Could you check a few things on this model? Use its own coordinates, in mm. A direction names the side the tool comes from. Round coordinates to 2 decimals unless told otherwise and drop trailing zeros. Order: outer loops, then holes, each group sorted by start corner. A loop starts at its lowest first (then second) coordinate and runs counter-clockwise, first axis right, second up. Notation, with made-up numbers: M 43,80.25 L 71,80.25 A24 cw 71,112.25 Z; hole C 39,62 d7. An arc over 180 degrees is marked long. Write each question's results on one line, items separated by ' | '. Start each with the question number.
1. Suppose I cut it at A-A on y = 946. Write out the boundary of the cut face in (x, z).
2. For faces 4 (the flat face through (-452, 553, 0)), 5 (the flat face through (-30, 276, 20)), which set-ups out of +Z, -Z, +X, -X, +Y, -Y let a thin tool reach every point of the face, with its end or its side?
3. Suppose I cut it at C-C on z = 28. Write out the boundary of the cut face in (x, y), and give its area (3 significant figures).
4. Suppose I cut it at B-B on x = -356.5. Write out the boundary of the cut face in (y, z).
5. We'd pull the mould along X, two halves only. Please class faces 1 (the flat face through (-870, 816, 20)), 2 (the flat face through (-19, 593, 50)), 3 (the flat face through (0, 542, 20)): released by +X, released by -X, zero draft, split by the parting line, or undercut.
6. I'm going to push flat-ended pins straight in: pin 1 (6 mm diameter, centred on x = -301, z = 50, fed in from +Y); pin 2 (5 mm diameter, centred on y = 542, z = 45, fed in from -X); pin 3 (6 mm diameter, centred on x = -693.5, z = 42.5, fed in from -Y); pin 4 (8 mm diameter, centred on y = 294, z = 45, fed in from -X). Where does each tip first touch, or does it pass through?
7. Please list where these lines run through material, in increasing order: L1, parallel to X at y = 1014, z = 35.5; L2, parallel to Y at x = -77, z = 37.5; L3, parallel to X at y = 364, z = 41.5.
from build123d import *

# Parameters (mm, degrees)
SKETCH1_W           = 900
SKETCH1_H           = 1100
SKETCH1_W_2         = 840
SKETCH1_H_2         = 1040
BOSS_EXTRUDE1_DEPTH = 50
FILLET1_R           = 10
SKETCH2_W           = 50
SKETCH2_H           = 1100
SKETCH2_W_2         = 868
SKETCH2_H_2         = 40
BOSS_EXTRUDE2_DEPTH = 60
FILLET2_R           = 10


with BuildPart() as part:
    # Sketch1 → Boss-Extrude1 (new body)
    with BuildSketch(Plane.XY):
        with Locations((-450, 550)):
            Rectangle(SKETCH1_W, SKETCH1_H)
        with Locations((-450, 550)):
            Rectangle(SKETCH1_W_2, SKETCH1_H_2, mode=Mode.SUBTRACT)
    extrude(amount=BOSS_EXTRUDE1_DEPTH)

    # Fillet1
    fillet1_edges = [part.edges().sort_by_distance(p)[0] for p in [
        (-900, 550, 50),
        (-450, 0, 50),
        (-450, 30, 50),
        (-30, 550, 50),
        (-450, 1070, 50),
        (-870, 550, 50),
        (0, 550, 50),
        (-450, 1100, 50),
    ]]
    fillet(fillet1_edges, radius=FILLET1_R)

    # Sketch2 → Boss-Extrude2 (add)
    with BuildSketch(Plane.XY):
        with Locations((-450, 550)):
            Rectangle(SKETCH2_W, SKETCH2_H)
        with Locations((-450, 550)):
            Rectangle(SKETCH2_W_2, SKETCH2_H_2)
    extrude(amount=BOSS_EXTRUDE2_DEPTH)

    # Fillet2
    fillet2_edges = [part.edges().sort_by_distance(p)[0] for p in [
        (-450, 0, 60),
        (-475, 265, 60),
        (-679.5, 530, 60),
        (-884, 550, 60),
        (-679.5, 570, 60),
        (-475, 835, 60),
        (-450, 1100, 60),
        (-425, 835, 60),
        (-220.5, 570, 60),
        (-16, 550, 60),
        (-220.5, 530, 60),
        (-425, 265, 60),
    ]]
    fillet(fillet2_edges, radius=FILLET2_R - 0.0001)  # a hair under: the kernel refuses the full size


solid = part.part
Filled sheet:
1) outline: M -900,0 L -870,0 L -870,40 A10 ccw -880,50 L -890,50 A10 ccw -900,40 Z; M -475,0 L -425,0 L -425,50 A10 ccw -435,60 L -465,60 A10 ccw -475,50 Z; M -30,0 L 0,0 L 0,40 A10 ccw -10,50 L -20,50 A10 ccw -30,40 Z
2) face 4: -Z, +X, -X, +Y, -Y | face 5: +Z, -Z
3) outline: M -900,0 L 0,0 L 0,1100 L -900,1100 Z; hole M -870,30 L -475,30 L -475,530 L -870,530 Z; hole M -870,570 L -475,570 L -475,1070 L -870,1070 Z; hole M -425,30 L -30,30 L -30,530 L -425,530 Z; hole M -425,570 L -30,570 L -30,1070 L -425,1070 Z | area: 200,000 mm^2
4) outline: M 0,0 L 30,0 L 30,40 A10 ccw 20,50 L 10,50 A10 ccw 0,40 Z; M 530,0 L 570,0 L 570,50 A10 ccw 560,60 L 540,60 A10 ccw 530,50 Z; M 1070,0 L 1100,0 L 1100,40 A10 ccw 1090,50 L 1080,50 A10 ccw 1070,40 Z
5) face 1: undercut | face 2: zero draft | face 3: released by +X
6) pin 1: stops at y = 1097.14 | pin 2: stops at x = -899.68 | pin 3: stops at y = 0 | pin 4: stops at x = -899.95
7) L1: x = -900 to -870, -475 to -425, -30 to 0 | L2: y = 0 to 30, 530 to 570, 1070 to 1100 | L3: x = -899.89 to -870.11, -475 to -425, -29.89 to -0.11
